Geometry: final body of the model. Coordinates: model frame, mm. A direction names the side the tool comes from. Give positions to 0.01 mm unless a question says otherwise; leave off trailing zeros. Loops run counter-clockwise (first coordinate to the right, second up) from the corner with the lowest first, then second, coordinate; pieces in that order, holes last.
from build123d import *

# Parameters (mm, degrees)
SKETCH1_R           = 75.5
BOSS_EXTRUDE1_DEPTH = 10
CUT_EXTRUDE1_START  = -10
SKETCH2_R           = 11
CUT_EXTRUDE1_DEPTH  = 5
SKETCH3_R           = 8
CUT_EXTRUDE2_DEPTH  = 107.890130508
SKETCH5_R           = 2.0828
CUT_EXTRUDE4_DEPTH  = 12.7
CIRPATTERN2_COUNT   = 3
CUT_EXTRUDE5_DEPTH  = 108.240384344
CIRPATTERN3_COUNT   = 6
CUT_EXTRUDE6_DEPTH  = 108.240384344
CIRPATTERN4_COUNT   = 3


with BuildPart() as part:
    # Sketch1 → Boss-Extrude1 (new body)
    with BuildSketch(Plane.XY):
        Circle(SKETCH1_R)
    extrude(amount=BOSS_EXTRUDE1_DEPTH)

    # Sketch2 → Cut-Extrude1 (cut)
    with BuildSketch(Plane.XY.offset(10).offset(CUT_EXTRUDE1_START)):
        Circle(SKETCH2_R)
    extrude(amount=CUT_EXTRUDE1_DEPTH, mode=Mode.SUBTRACT)

    # Sketch3 → Cut-Extrude2 (cut, through all)
    with BuildSketch(Plane(origin=(0, 0, 5), x_dir=(-1, 0, 0), z_dir=(0, 0, -1))):
        Circle(SKETCH3_R)
    extrude(amount=-CUT_EXTRUDE2_DEPTH, mode=Mode.SUBTRACT)

    # Sketch5 → Cut-Extrude4 (cut)
    with BuildSketch(Plane(origin=(0, 75.5, 0), x_dir=(1, 0, 0), z_dir=(0, 1, 0))):
        with Locations(Location((0, -5.08, 0), (0, 0, 270))):
            Circle(SKETCH5_R)
    cut_extrude4 = extrude(amount=-CUT_EXTRUDE4_DEPTH, mode=Mode.SUBTRACT)

    # CirPattern2: Cut-Extrude4 ×3 about axis
    cirpattern2_axis = Axis((0, 0, 0), (0, 0, 1))
    for i in range(1, CIRPATTERN2_COUNT):
        add(cut_extrude4.rotate(cirpattern2_axis, i * 360 / CIRPATTERN2_COUNT), mode=Mode.SUBTRACT)

    # Sketch6 → Cut-Extrude5 (cut, through all)
    with BuildSketch(Plane(origin=(0, 0, 0), x_dir=(-1, 0, 0), z_dir=(0, 0, -1))):
        with BuildLine():
            Line((-25.430689936, 50.397247041), (-8.993552206, 21.927289361))
            ThreePointArc((-8.993552206, 21.927289361), (0, 23.7), (8.993552206, 21.927289361))
            Line((8.993552206, 21.927289361), (25.430689936, 50.397247041))
            ThreePointArc((25.430689936, 50.397247041), (13.070537583, 54.915968054), (3.6e-08, 56.45))
            ThreePointArc((3.6e-08, 56.45), (-13.070537548, 54.915968062), (-25.430689936, 50.397247041))
        make_face()
        with BuildLine():
            ThreePointArc((3.6e-08, 56.45), (13.070537583, 54.915968054), (25.430689936, 50.397247041))
            Line((25.430689936, 50.397247041), (28.61021379, 55.9043439))
            ThreePointArc((28.61021379, 55.9043439), (17.78253642, 60.229738489), (6.341879371, 62.478960987))
            ThreePointArc((6.341879371, 62.478960987), (4.375151569, 58.197766982), (3.6e-08, 56.45))
        make_face()
        with BuildLine():
            Line((-28.61021379, 55.9043439), (-25.430689936, 50.397247041))
            ThreePointArc((-25.430689936, 50.397247041), (-13.070537548, 54.915968062), (3.6e-08, 56.45))
            ThreePointArc((3.6e-08, 56.45), (-4.375151542, 58.197766957), (-6.341879371, 62.478960987))
            ThreePointArc((-6.341879371, 62.478960987), (-17.78253642, 60.229738489), (-28.61021379, 55.9043439))
        make_face()
    cut_extrude5 = extrude(amount=-CUT_EXTRUDE5_DEPTH, mode=Mode.SUBTRACT)

    # CirPattern3: Cut-Extrude5 ×6 about axis
    cirpattern3_axis = Axis((0, 0, 0), (0, 0, 1))
    for i in range(1, CIRPATTERN3_COUNT):
        add(cut_extrude5.rotate(cirpattern3_axis, i * 360 / CIRPATTERN3_COUNT), mode=Mode.SUBTRACT)

    # Sketch8 → Cut-Extrude6 (cut, through all)
    with BuildSketch(Plane(origin=(0, 0, 0), x_dir=(-1, 0, 0), z_dir=(0, 0, -1))):
        with BuildLine():
            ThreePointArc((-57.279307102, 25.747251851), (-48.887134044, 28.225), (-50.937427732, 36.731709136))
            ThreePointArc((-50.937427732, 36.731709136), (-54.386395358, 31.4), (-57.279307102, 25.747251851))
        make_face()
    cut_extrude6 = extrude(amount=-CUT_EXTRUDE6_DEPTH, mode=Mode.SUBTRACT)

    # CirPattern4: Cut-Extrude6 ×3 about axis
    cirpattern4_axis = Axis((0, 0, 5), (0, 0, -1))
    for i in range(1, CIRPATTERN4_COUNT):
        add(cut_extrude6.rotate(cirpattern4_axis, i * 360 / CIRPATTERN4_COUNT), mode=Mode.SUBTRACT)


solid = part.part
Item 1: Draft query along X for faces 1 (the face through (-43.15, -45.63, 4.93)), 2 (the face through (72.014, 22.678, 4.93)), 3 (the face through (-1, -16, 0)). Return one class per face: +X half, -X half, draft (parallel to the pull), parting line (faces both ways), or undercut.
Values follow:
face 1: undercut
face 2: parting line
face 3: draft
Item 2: Set-up query: faces 4 (the face through (20.46, -11.96, 4.93)), 5 (the face through (0, 62.8, 5)), 6 (the face through (-2, -8, 5)), 7 (the face through (54.37, -31.43, 5.05)). Return all of +Z, -Z, +X, -X, +Y, -Y with unobstructed straight access to the full face (end or side cutting, diameter ignored); none if empty.
Values follow:
face 4: +Z, -Z
face 5: +Y
face 6: -Z
face 7: none
Item 3: Section query A-A on y = 0. Return loops of the section in (x, z), plus the area to 3 significant figures.
Values follow:
outline: (-75.5, 0) - (-11, 0) - (-11, 5) - (-8, 5) - (-8, 10) - (-75.5, 10) - close; (8, 5) - (11, 5) - (11, 0) - (75.5, 0) - (75.5, 10) - (8, 10) - close
area: 1,320 mm2
Item 4: Pin query (flat end, axial travel): pin 1 (3 mm diameter, centred on x = -48, z = 5.5, fed in from +Y); pin 2 (1.9 mm diameter, centred on x = 58, z = 5.5, fed in from +Y); pin 3 (3 mm diameter, centred on x = 46, z = 7.5, fed in from +Y). Return the tip coordinate at first contact, or that it passes through.
Values follow:
pin 1: stops at y = 59.48
pin 2: stops at y = 49.45
pin 3: stops at y = 60.99
Item 5: Ray query, probe 1 along Y at (x, z) = (0.5, 7.5); probe 2 along Y at (x, z) = (-36, 3.25) (3 decimals); probe 3 along Y at (x, z) = (-5, 7) (3 decimals). Return the intervals inside material, ascending.
Values follow:
probe 1: y = -75.5 to -62.8, -23.69 to -7.98, 7.98 to 23.69, 56.47 to 75.5
probe 2: y = -66.365 to -51.457, -3.175 to 3.175, 51.457 to 66.365
probe 3: y = -75.334 to -62.601, -23.167 to -6.245, 6.245 to 23.167, 58.886 to 75.334
